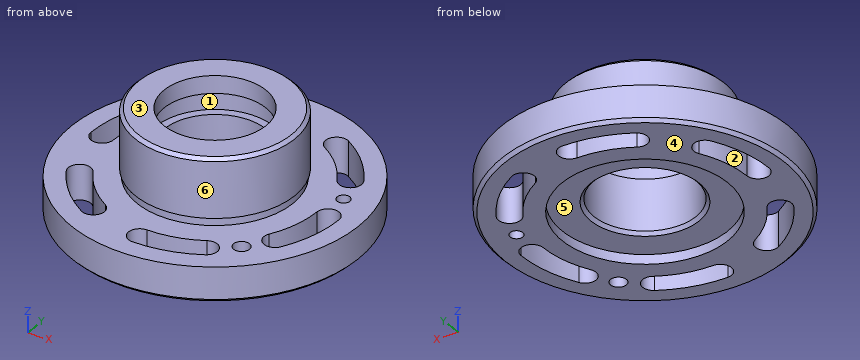
from build123d import *

# Parameters (mm, degrees)
SKETCH_1_R               = 90
EXTRUDE_1_DEPTH          = 22
SKETCH_2_R               = 50
EXTRUDE_2_DEPTH          = 42
SKETCH_3_OUTSIDE_W       = 234.496
SKETCH_3_OUTSIDE_H       = 234.496
SKETCH_3_OUTSIDE_R       = 49
CUT_EXTRUDE_1_DEPTH      = 5
SKETCH_4_R               = 32
CUT_EXTRUDE_2_DEPTH      = 143.464030548
CUT_EXTRUDE_START        = -24
SKETCH_5_R               = 37
CUT_EXTRUDE_3_DEPTH      = 13
SKETCH_6_R               = 52
CUT_EXTRUDE_4_DEPTH      = 6
CHAMFER_1_SIZE           = 2
CUT_EXTRUDE_5_DEPTH      = 135.029847422
PATTERN_CIRCULAR_1_COUNT = 6
F_10_0MM_2_D             = 10
F_8_0MM_1_D              = 8


with BuildPart() as part:
    # 草图1 → 凸台-拉伸1 (new body)
    with BuildSketch(Plane.XY):
        Circle(SKETCH_1_R)
    extrude(amount=EXTRUDE_1_DEPTH)

    # 草图2 → 凸台-拉伸2 (add)
    with BuildSketch(Plane.XY.offset(22)):
        with Locations(Location((0, 0, 0), (0, 0, 180))):
            Circle(SKETCH_2_R)
    extrude(amount=EXTRUDE_2_DEPTH)

    # 草图3 outside → 切除-拉伸1 (cut)
    with BuildSketch(Plane.XY.offset(22)):
        Rectangle(SKETCH_3_OUTSIDE_W, SKETCH_3_OUTSIDE_H)
        Circle(SKETCH_3_OUTSIDE_R, mode=Mode.SUBTRACT)
    extrude(amount=CUT_EXTRUDE_1_DEPTH, mode=Mode.SUBTRACT)

    # 草图4 → 切除-拉伸2 (cut, through all)
    with BuildSketch(Plane.XY.offset(64)):
        Circle(SKETCH_4_R)
    extrude(amount=-CUT_EXTRUDE_2_DEPTH, mode=Mode.SUBTRACT)

    # 草图5 → 切除-拉伸3 (cut)
    with BuildSketch(Plane.XY.offset(64).offset(CUT_EXTRUDE_START)):
        with Locations(Location((0, 0, 0), (0, 0, 180))):
            Circle(SKETCH_5_R)
    extrude(amount=CUT_EXTRUDE_3_DEPTH, mode=Mode.SUBTRACT)

    # 草图6 → 切除-拉伸4 (cut)
    with BuildSketch(Plane(origin=(0, 0, 0), x_dir=(-1, 0, 0), z_dir=(0, 0, -1))):
        Circle(SKETCH_6_R)
    extrude(amount=-CUT_EXTRUDE_4_DEPTH, mode=Mode.SUBTRACT)

    # 倒角1
    chamfer_1_edges = [part.edges().sort_by_distance(p)[0] for p in [
        (-90, 0, 0),
        (-32, 0, 6),
        (50, 0, 64),
    ]]
    chamfer(chamfer_1_edges, length=CHAMFER_1_SIZE)

    # 草图7 → 切除-拉伸5 (cut, through all)
    with BuildSketch(Plane.XY.offset(22)):
        with BuildLine():
            ThreePointArc((0, 78), (-20.187885518, 75.342214451), (-39, 67.549981495))
            ThreePointArc((-39, 67.549981495), (-41.562177826, 57.987803669), (-32, 55.425625842))
            ThreePointArc((-32, 55.425625842), (-16.564418887, 61.819252883), (0, 64))
            ThreePointArc((0, 64), (7, 71), (0, 78))
        make_face()
    cut_extrude_5 = extrude(amount=-CUT_EXTRUDE_5_DEPTH, mode=Mode.SUBTRACT)

    # 阵列(圆周)1: 切除-拉伸5 ×6 about axis
    pattern_circular_1_axis = Axis((0, 0, 0), (0, 0, 1))
    for i in range(1, PATTERN_CIRCULAR_1_COUNT):
        add(cut_extrude_5.rotate(pattern_circular_1_axis, i * 360 / PATTERN_CIRCULAR_1_COUNT), mode=Mode.SUBTRACT)

    # Ø10.0mm 暗销孔2 (through all)
    with Locations(Plane.XY.offset(22)):
        with Locations((50.204581464, -50.204581464)):
            Hole(F_10_0MM_2_D / 2)

    # Ø8.0mm 暗销孔1 (through all)
    with Locations(Plane.XY.offset(22)):
        with Locations((68.580733667, 18.376152202)):
            Hole(F_8_0MM_1_D / 2)


solid = part.part
Could you check a few things on this model? Use its own coordinates, in mm. Face numbers are marked on the shaded views. A direction names the side the tool comes from. Round coordinates to 2 decimals unless told otherwise and drop trailing zeros. Loops run counter-clockwise (first coordinate to the right, second up) from the corner with the lowest first, then second, coordinate; pieces in that order, holes last. Notation, with made-up numbers: (-12.5, 22) - (12.5, 22) arc R30 ccw to (12.5, 56) - close; hole circle Ø5 at (22, 21). An arc over 180 degrees is marked (long way). Write item = value, one per line.
1) I need wall thicknesses on line 1 along X through (y, z) = (6, 9.5); line 2 along X through (y, z) = (-0.5, 18); line 3 along Y through (x, z) = (52.5, 3). Which ranges of each line are inside material? Lowest first, please. Write a range as from..to.
Computed:
line_1 = -89.8..-77.77, -63.72..-31.43, 31.43..67.39, 74.61..89.8
line_2 = -90..-77.98, -64.02..-32, 32..64, 78..90
line_3 = -73.1..-54.65, -45.76..36.6, 57.69..73.1
2) Imagine slicing it at B-B (y = -11). Give the number of separate pieces and of enclosed holes in the cut face, and give its area (3 significant figures).
Computed:
separate_pieces = 3
enclosed_holes = 0
area = 3,460 mm2
3) Imagine slicing it at D-D (z = 49). Please give me the cut outline in (x, y), and give its area (3 significant figures).
Computed:
outline = circle Ø100 at (0, 0); hole circle Ø74 at (0, 0)
area = 3,550 mm2
4) Imagine slicing it at A-A (z = 34). Please give me the cut outline in (x, y).
Computed:
outline = circle Ø100 at (0, 0); hole circle Ø64 at (0, 0)
5) I'm going to push flat-ended pins straight in: P1, Ø10, axis at y = 61.5, z = 17.5, coming from the +X side; P2, Ø6, axis at x = 63, z = 17, coming from the -Y side; P3, Ø2, axis at y = -41, z = 41.5, coming from the -X side; P4, Ø6.5, axis at x = 68.58, y = 18.38, coming from the +Z side. Where does each tip first touch, or does it pass through?
Computed:
P1 = 70.06
P2 = -67.08
P3 = -30
P4 = through
6) If we mould it in two halves opening along X, with no side actions, what happens to the marked faces 4, 5 and 6? For each: pulls with the +X half, pulls with the -X half, needs draft (parallel to the pull), parting line crosses it, or undercut.
Computed:
face_4 = needs draft
face_5 = undercut
face_6 = parting line crosses it
7) On a 3-axis mill with a long thin cutter (end or side, diameter ignored), from which of +Z, -Z, +X, -X, +Y, -Y can I reach the whole of each face in a straight line? I mean the marked faces 1, 2 and 3. Say none if no direction works.
Computed:
face_1 = none
face_2 = +Z, -Z
face_3 = +Z, +X, -X, +Y, -Y
